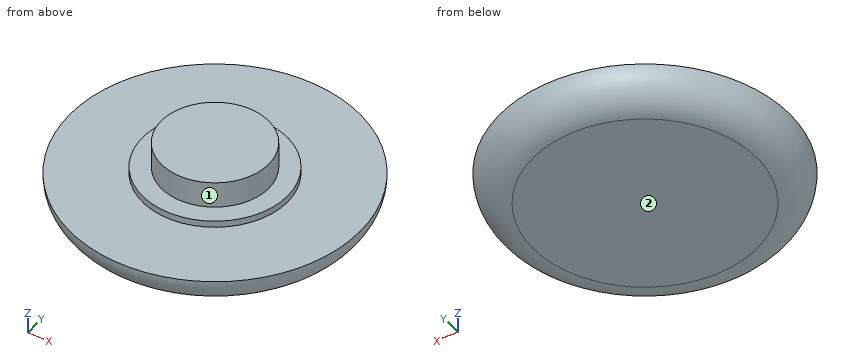
```python
from build123d import *

# Parameters (mm, degrees)
F0_R     = 11
F0_R_2   = 5.5
F1_DEPTH = 2.5
F0_R_3   = 4.075
F2_DEPTH = 3
F3_DEPTH = 5
F4_R     = 2.49999


# Not quite as in the source:
# - a fillet or chamfer is up to 0.001 mm smaller than in the source, because OpenCascade refuses the exact size


with BuildPart() as f1:
    # F0 (on Top) → F1 (new body)
    with BuildSketch(Plane.XY):
        with Locations((-41.2729866803, 41.5038391948)):
            Circle(F0_R)
        with Locations((-41.2729866803, 41.5038391948)):
            Circle(F0_R_2, mode=Mode.SUBTRACT)
    extrude(amount=F1_DEPTH)

    # F0 (on Top) → F2 (join)
    with BuildSketch(Plane.XY):
        with Locations((-41.2729866803, 41.5038391948)):
            Circle(F0_R_2)
        with Locations((-41.2729866803, 41.5038391948)):
            Circle(F0_R_3, mode=Mode.SUBTRACT)
    extrude(amount=F2_DEPTH)

    # F0 (on Top) → F3 (join)
    with BuildSketch(Plane.XY):
        with Locations((-41.2729866803, 41.5038391948)):
            Circle(F0_R_3)
    extrude(amount=F3_DEPTH)

    # F4 (radius 2.5 in the source; OpenCascade refuses exactly that, so slightly less here)
    f4_edges = [f1.edges().sort_by_distance(p)[0] for p in [
        (-52.272987, 41.503839, 0),
    ]]
    fillet(f4_edges, radius=F4_R)


solid = f1.part
```
Here's how the part is built. I have some questions about the finished solid (model axes, mm). Face numbers are marked on the shaded views. A direction names the side the tool comes from. Coordinates: 2 decimals unless noted, no trailing zeros. Order: outer loops, then holes, each group sorted by start corner. A loop starts at its lowest first (then second) coordinate and runs counter-clockwise, first axis right, second up. Notation, with made-up numbers: M -20.5,19.25 L 9.5,19.25 A21 cw 9.5,28.25 Z; hole C 21.25,-18.5 d3. An arc over 180 degrees is marked long. Answer as a JSON object with one key per item and string values. Group by question number.
(1) Suppose I cut it at B-B, the plane z = 3.75. Please give me the cut outline in (x, y) (3 decimals), then the cut area to 3 significant figures.
(2) For pin 1 (5 mm diameter, centred on x = -36, y = 35, fed in from +Z); pin 2 (1 mm diameter, centred on x = -37.5, z = 1.5, fed in from -Y); pin 3 (1 mm diameter, centred on y = 33.5, z = 4, fed in from +X), each with a flat end and sliding along its axis, tell me the tip position at first contact or that it passes through.
(3) I need wall thicknesses on probe 1 along Z at (x, y) = (-48.25, 44); probe 2 along Z at (x, y) = (-40.5, 46.25); probe 3 along X at (y, z) = (32.75, 1.55). Which ranges of each line are inside material? Lowest first, please.
(4) Which directions (+Z, -Z, +X, -X, +Y, -Y) give clear straight access to the entire face, cutting with the end or side of a thin tool? Please do the marked faces 1 and 2.
(5) Suppose I cut it at A-A, the plane z = 0.35. Please give me the cut outline in (x, y), then the cut area to 3 significant figures.
Values found:
{
 "1": {"outline": "C -41.273,41.504 d8.15", "area": "52.2 mm^2"},
 "2": {"pin 1": "stops at z = 2.5", "pin 2": "stops at y = 31.14", "pin 3": "passes through"},
 "3": {"probe 1": "z = 0 to 2.5", "probe 2": "z = 0 to 3", "probe 3": "x = -47.62 to -34.93"},
 "4": {"face 1": "+Z", "face 2": "-Z, +X, -X, +Y, -Y"},
 "5": {"outline": "C -41.27,41.5 d19.55", "area": "300 mm^2"}
}
